Can you work these out from the model? Positions are in its coordinate system, mm. Face numbers are marked on the shaded views. Give positions to 0.01 mm unless a question says otherwise; leave off trailing zeros. Loops run counter-clockwise (first coordinate to the right, second up) from the corner with the lowest first, then second, coordinate; pieces in that order, holes last. Notation, with made-up numbers: (70, 60.25) - (128, 60.25) arc R15 cw to (128, 85.25) - close; hole circle Ø5 at (49, 89.25). An arc over 180 degrees is marked (long way). Answer in a Markdown table with one row per item.
from build123d import *

# Parameters (mm, degrees)
F1_DEPTH = 3
F2_DEPTH = 15
F3_R     = 1.6
F4_DEPTH = 25
F5_R     = 1.75
F6_DEPTH = 25
F5_R_2   = 4.5
F5_R_3   = 3.5
F7_DEPTH = 1
F8_SIZE2 = 2.1
F8_SIZE  = 3.5


with BuildPart() as f1:
    # F0 (on Top) → F1 (new body)
    with BuildSketch(Plane.XY):
        Polygon((-4.5, -12.5), (7.5, 9.5), (-4.5, 9.5), align=None)
    extrude(amount=F1_DEPTH)

    # F0 (on Top) → F2 (join)
    with BuildSketch(Plane.XY):
        Polygon((7.5, 9.5), (7.5, 12.5), (-7.5, 12.5), (-7.5, -12.5), (-4.5, -12.5), (-4.5, 9.5), align=None)
    extrude(amount=F2_DEPTH)

    # F3 (on face) → F4 (cut)
    with BuildSketch(Plane(origin=(-7.5, 0, 0), x_dir=(0, -1, 0), z_dir=(-1, 0, 0))):
        with Locations((5.8420459367, 9.0217133984)):
            Circle(F3_R)
    extrude(amount=-F4_DEPTH, mode=Mode.SUBTRACT)

    # F5 (on face) → F6 (cut)
    with BuildSketch(Plane.XZ.offset(-9.5)):
        with Locations((0.5, 9)):
            Circle(F5_R)
    extrude(amount=-F6_DEPTH, mode=Mode.SUBTRACT)

    # F5 (on face) → F7 (join)
    with BuildSketch(Plane.XZ.offset(-9.5)):
        with Locations((0.5, 9)):
            Circle(F5_R_2)
        with Locations((0.5, 9)):
            Circle(F5_R_3, mode=Mode.SUBTRACT)
        with Locations((0.5, 9)):
            Circle(F5_R_3)
        with Locations((0.5, 9)):
            Circle(F5_R, mode=Mode.SUBTRACT)
    extrude(amount=F7_DEPTH)

    # F8
    f8_edges = [f1.edges().sort_by_distance(p)[0] for p in [
        (-1.25, 8.5, 9),
    ]]
    f8_side = f1.faces().sort_by_distance((-1.25, 9, 9))[0]
    chamfer(f8_edges, length=F8_SIZE, length2=F8_SIZE2, reference=f8_side)


solid = f1.part
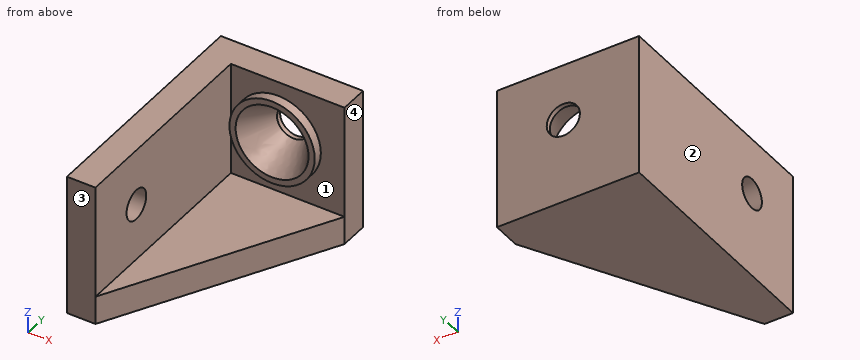
Q1. Imagine slicing it at B-B, the plane z = 1.5. Write out the boundary of the cut face in (x, y), and give its area (3 significant figures).
Checked values:
| item | result |
|---|---|
| outline | (-7.5, -12.5) - (-4.5, -12.5) - (7.5, 9.5) - (7.5, 12.5) - (-7.5, 12.5) - close |
| area | 243 mm² |
Q2. If we mould it in two halves opening along X, with no side actions, what happens to the marked faces 1, 2, 3 and 4? For each: released by +X, released by -X, zero draft, split by the parting line, or undercut.
Checked values:
| item | result |
|---|---|
| face 1 | undercut |
| face 2 | released by -X |
| face 3 | zero draft |
| face 4 | released by +X |
Q3. Imagine slicing it at D-D, the plane y = 1. Write out the boundary of the cut face in (x, z), and give its area (3 significant figures).
Checked values:
| item | result |
|---|---|
| outline | (-7.5, 0) - (2.86, 0) - (2.86, 3) - (-4.5, 3) - (-4.5, 15) - (-7.5, 15) - close |
| area | 67.1 mm² |
Q4. Imagine slicing it at C-C, the plane x = -6.5. Write out the boundary of the cut face in (y, z).
Checked values:
| item | result |
|---|---|
| outline | (-12.5, 0) - (12.5, 0) - (12.5, 15) - (-12.5, 15) - close; hole circle Ø3.2 at (-5.84, 9.02) |
Q5. For pin 1 (8 mm diameter, centred on y = -9.5, z = 13, fed in from +X); pin 2 (3 mm diameter, centred on x = -1, y = 2, fed in from +Z); pin 3 (4 mm diameter, centred on x = 5, z = 3, fed in from -Y); pin 4 (1.5 mm diameter, centred on x = -0.5, y = -9.5, fed in from -Z) (1 decimal), each with a flat end and sliding along its axis, tell me the tip position at first contact or that it passes through.
Checked values:
| item | result |
|---|---|
| pin 1 | stops at x = -4.5 |
| pin 2 | stops at z = 3 |
| pin 3 | stops at y = 1.25 |
| pin 4 | passes through |
Q6. Imagine slicing it at A-A, the plane y = -4.75. Write out the boundary of the cut face in (x, z).
Checked values:
| item | result |
|---|---|
| outline | (-7.5, 0) - (-0.27, 0) - (-0.27, 3) - (-4.5, 3) - (-4.5, 7.85) - (-7.5, 7.85) - close; (-7.5, 10.19) - (-4.5, 10.19) - (-4.5, 15) - (-7.5, 15) - close |
Q7. If I drill on line 1 (X direction, y = 12.35, z = 9); line 2 (Z direction, x = -4.75, y = -5.75); line 3 (X direction, y = -10.25, z = 4.75), over which ranges is the centre line in solid material (lowest first)? Write a range as [from, to].
Checked values:
| item | result |
|---|---|
| line 1 | x = [-7.5, -1.25], [2.25, 7.5] |
| line 2 | z = [0, 7.42], [10.62, 15] |
| line 3 | x = [-7.5, -4.5] |
